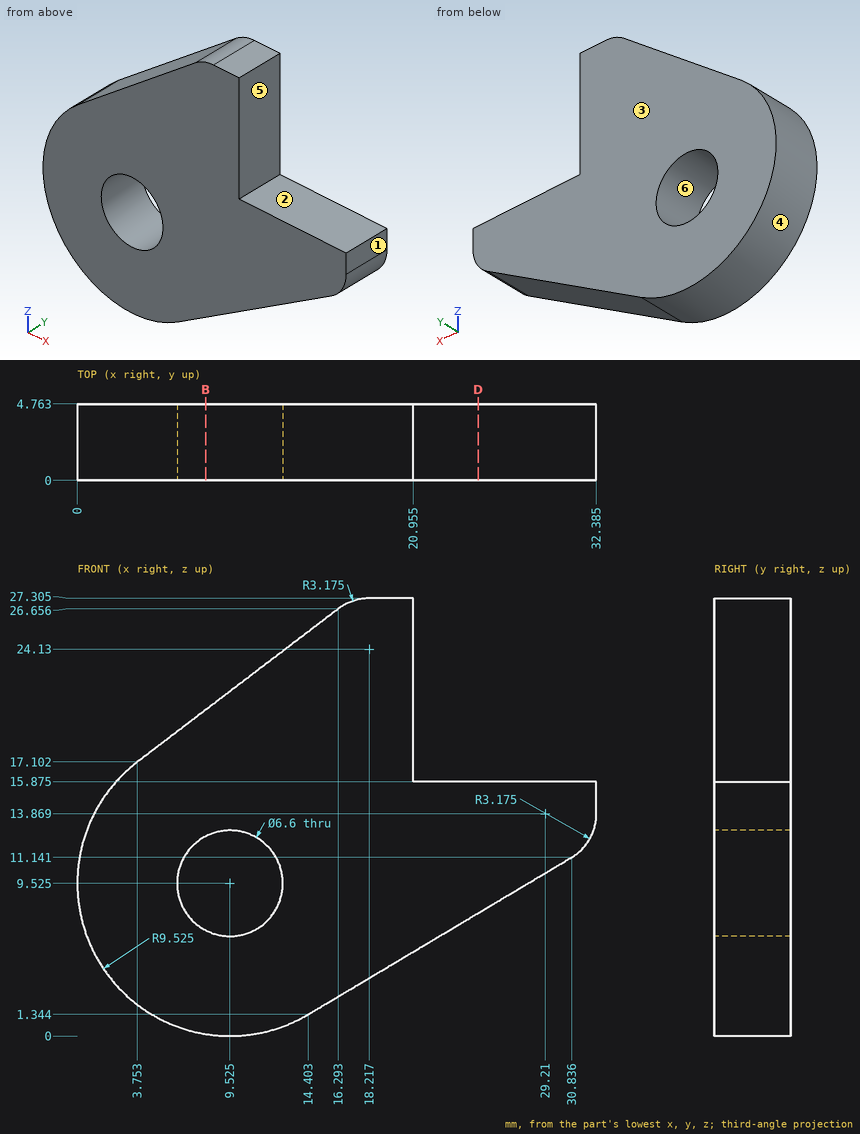
Design review of the part shown in the three views and the two pictorial views. Dimensions are in mm from the part's minimum x, y and z. A direction names the side the tool comes from. Round coordinates to 2 decimals unless told otherwise and drop trailing zeros. Order: outer loops, then holes, each group sorted by start corner. A loop starts at its lowest first (then second) coordinate and runs counter-clockwise, first axis right, second up. Notation, with made-up numbers: (69, -21) -> (110, -21) arc R29 ccw to (110, 1) -> close; hole circle Ø1 at (65, 63.5). An arc over 180 degrees is marked (long way). Write item = value, one per line. Start each with the question number.
1) The part is to be moulded in two halves that separate along X. For the marked faces 3, 4, 5 and 6, say which applies: +X half, -X half, draft (parallel to the pull), parting line (faces both ways), or undercut.
2) To check wall thickness, follow line 1 (X direction, y = 1.6, z = 11) (1 decimal); line 2 (X direction, y = 2.5, z = 9.75) (1 decimal); line 3 (X direction, y = 0.45, z = 15) (1 decimal). State the ranges of each line that lie inside material, in increasing order. Write a range as from..to.
3) Take a section at D-D on x = 25. State the section outline as (y, z) points (1 decimal), plus the area to 3 significant figures.
4) Insertion check: pin 1 (3 mm diameter, centred on x = 15.5, z = 24.5, fed in from -Y); pin 2 (1.4 mm diameter, centred on x = 26.5, y = 3.5, fed in from +Z) (1 decimal). Each pin has a flat end and moves straight along its axis. Give the tip position at first contact, or say it passes through.
5) Take a section at B-B on x = 8. State the section outline as (y, z) points.
6) Tool access review of the marked faces 1 and 2: name each direction out of +Z, -Z, +X, -X, +Y, -Y from which nothing blocks a thin tool from reaching the whole face with its end or side.
Verdict:
q1.face_3 = draft
q1.face_4 = parting line
q1.face_5 = +X half
q1.face_6 = undercut
q2.line_1 = 0.1..6.6, 12.5..30.6
q2.line_2 = 0..6.2, 12.8..28.5
q2.line_3 = 1.7..32.4
q3.outline = (0, 7.7) -> (4.8, 7.7) -> (4.8, 15.9) -> (0, 15.9) -> close
q3.area = 39.1 mm2
q4.pin_1 = 0
q4.pin_2 = 15.9
q5.outline = (0, 0.12) -> (4.76, 0.12) -> (4.76, 6.6) -> (0, 6.6) -> close; (0, 12.45) -> (4.76, 12.45) -> (4.76, 20.34) -> (0, 20.34) -> close
q6.face_1 = +Z, -Z, +X, +Y, -Y
q6.face_2 = +Z, +X, +Y, -Y
